The listing builds one solid part. Answer for the finished solid, in the listing's coordinates (mm). Face numbers are marked on the shaded views. A direction names the side the tool comes from. Round coordinates to 2 decimals unless told otherwise and drop trailing zeros. Write each loop counter-clockwise with the first axis right and the second up, starting at its lowest first coordinate (ties: lowest second). Pieces come first, ordered by that corner, then holes. Notation, with made-up numbers: (32.5, 73) - (74.5, 73) arc R11 cw to (74.5, 84) - close; hole circle Ø10 at (-27.75, -20). An arc over 180 degrees is marked (long way). Answer in a Markdown table with one row per item.
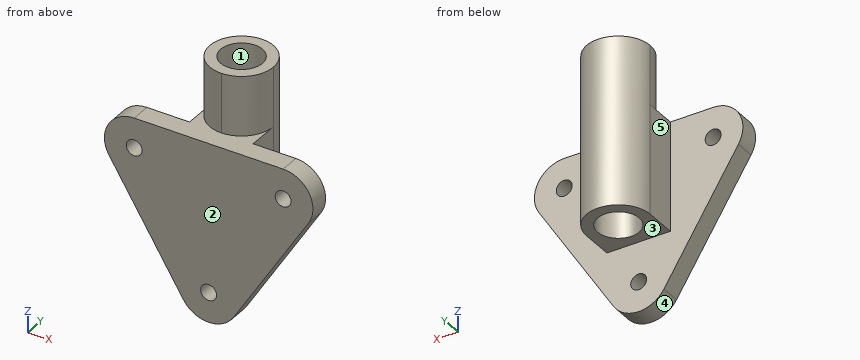
from build123d import *

# Parameters (mm, degrees)
SKETCH2_R               = 4
BOSS_EXTRUDE1_DEPTH     = 10
BOSS_EXTRUDE2_DEPTH     = 85
SKETCH5_R               = 10.5
CUT_EXTRUDE1_DEPTH      = 36
CUT_EXTRUDE1_DEPTH_BACK = 86
CUT_EXTRUDE2_DEPTH      = 30


with BuildPart() as part:
    # Sketch2 → Boss-Extrude1 (new body)
    with BuildSketch(Plane(origin=(0, 0, 0), x_dir=(1, 0, 0), z_dir=(0, 1, 0))):
        with BuildLine():
            Line((-50.21997456, -52.0500159), (-12.71997456, 7.9499841))
            ThreePointArc((-12.71997456, 7.9499841), (0, 15), (12.71997456, 7.9499841))
            Line((12.71997456, 7.9499841), (50.21997456, -52.0500159))
            ThreePointArc((50.21997456, -52.0500159), (50.619637219, -67.271527986), (37.5, -75))
            Line((37.5, -75), (-37.5, -75))
            ThreePointArc((-37.5, -75), (-50.619637219, -67.271527986), (-50.21997456, -52.0500159))
        make_face()
        Circle(SKETCH2_R, mode=Mode.SUBTRACT)
        with Locations((-37.5, -60)):
            Circle(SKETCH2_R, mode=Mode.SUBTRACT)
        with Locations((37.5, -60)):
            Circle(SKETCH2_R, mode=Mode.SUBTRACT)
    extrude(amount=BOSS_EXTRUDE1_DEPTH)

    # Sketch4 → Boss-Extrude2 (add)
    with BuildSketch(Plane.XY.offset(20)):
        with BuildLine():
            Line((16, 26), (16, 10))
            Line((16, 10), (-16, 10))
            Line((-16, 10), (-16, 26))
            ThreePointArc((-16, 26), (0, 42), (16, 26))
        make_face()
    extrude(amount=BOSS_EXTRUDE2_DEPTH)

    # Sketch5 → Cut-Extrude1 (cut, two sides)
    with BuildSketch(Plane(origin=(0, 0, 20), x_dir=(-1, 0, 0), z_dir=(0, 0, -1))) as cut_extrude1_sk:
        with Locations((0, 26)):
            Circle(SKETCH5_R)
    extrude(amount=CUT_EXTRUDE1_DEPTH, mode=Mode.SUBTRACT)
    extrude(cut_extrude1_sk.sketch, amount=-CUT_EXTRUDE1_DEPTH_BACK, mode=Mode.SUBTRACT)

    # Sketch6 → Cut-Extrude2 (cut)
    with BuildSketch(Plane.XY.offset(105)):
        with BuildLine():
            ThreePointArc((16, 26), (11.313708518, 14.68629152), (5.5e-08, 10))
            Line((5.5e-08, 10), (16, 10))
            Line((16, 10), (16, 26))
        make_face()
        with BuildLine():
            ThreePointArc((5.5e-08, 10), (-11.31370848, 14.686291482), (-16, 26))
            Line((-16, 26), (-16, 10))
            Line((-16, 10), (5.5e-08, 10))
        make_face()
    extrude(amount=-CUT_EXTRUDE2_DEPTH, mode=Mode.SUBTRACT)


solid = part.part
(1) Section D-D (z = 2) is taken. Give the vertices of the cut face in (x, y).
Checked values:
| item | result |
|---|---|
| outline | (-18.94, 0) - (-3.46, 0) - (-3.46, 10) - (-18.94, 10) - close; (3.46, 0) - (18.94, 0) - (18.94, 10) - (3.46, 10) - close |
(2) Section B-B (y = 4) is taken. Give the vertices of the cut face in (x, z).
Checked values:
| item | result |
|---|---|
| outline | (-50.22, 52.05) - (-12.72, -7.95) arc R15 ccw to (12.72, -7.95) - (50.22, 52.05) arc R15 ccw to (37.5, 75) - (-37.5, 75) arc R15 ccw to start; hole circle Ø8 at (-37.5, 60); hole circle Ø8 at (0, 0); hole circle Ø8 at (37.5, 60) |
(3) Section A-A (z = 60) is taken. Give the vertices of the cut face in (x, y), and give its area (3 significant figures).
Checked values:
| item | result |
|---|---|
| outline | (-52.5, 0) - (-41.5, 0) - (-41.5, 10) - (-52.5, 10) - close; (-33.5, 0) - (33.5, 0) - (33.5, 10) - (16, 10) - (16, 26) arc R16 ccw to (-16, 26) - (-16, 10) - (-33.5, 10) - close; (41.5, 0) - (52.5, 0) - (52.5, 10) - (41.5, 10) - close; hole circle Ø21 at (0, 26) |
| area | 1,460 mm2 |
(4) Find the intervals of material crossed by line 1 (X direction, y = 3, z = 60); line 2 (Y direction, x = 0, z = 42.5); line 3 (Z direction, x = 37, y = 5), in increasing order.
Checked values:
| item | result |
|---|---|
| line 1 | x = -52.5 to -41.5, -33.5 to 33.5, 41.5 to 52.5 |
| line 2 | y = 0 to 15.5, 36.5 to 42 |
| line 3 | z = 30.9 to 56.03, 63.97 to 75 |
(5) Flat-ended cylindrical pins translate along their axes: pin 1 (8 mm diameter, centred on y = 7.5, z = 2.5, fed in from +X); pin 2 (9.5 mm diameter, centred on x = 5, y = 24.5, fed in from -Z); pin 3 (10 mm diameter, centred on x = 15, z = 22.5, fed in from +Y); pin 4 (10 mm diameter, centred on x = 28.5, z = 22.5, fed in from +Y). Find the tip coordinate at first contact, or state that the pin passes through.
Checked values:
| item | result |
|---|---|
| pin 1 | stops at x = 21.75 |
| pin 2 | passes through |
| pin 3 | stops at y = 38.49 |
| pin 4 | stops at y = 10 |
(6) For the marked faces 4 and 5, determine the directions among +Z, -Z, +X, -X, +Y, -Y from which every point of the face is accessible in a straight line to the end or side of a thin tool.
Checked values:
| item | result |
|---|---|
| face 4 | -Z, +Y, -Y |
| face 5 | +Z, -Z, -X, +Y |
(7) Section C-C (y = 30.5) is taken. Give the vertices of the cut face in (x, z).
Checked values:
| item | result |
|---|---|
| outline | (-15.35, 20) - (-9.49, 20) - (-9.49, 105) - (-15.35, 105) - close; (9.49, 20) - (15.35, 20) - (15.35, 105) - (9.49, 105) - close |
(8) For a pull along Y with two mould halves and no side action, classify the marked faces 1, 2 and 3 as pulls with the +Y half, pulls with the -Y half, needs draft (parallel to the pull), parting line crosses it, or undercut.
Checked values:
| item | result |
|---|---|
| face 1 | undercut |
| face 2 | pulls with the -Y half |
| face 3 | needs draft |
